Here's the drawing with two shaded views (mm, measured from the low corner). I have some questions. A direction names the side the tool comes from. Give positions to 0.01 mm unless a question says otherwise; leave off trailing zeros. Loops run counter-clockwise (first coordinate to the right, second up) from the corner with the lowest first, then second, coordinate; pieces in that order, holes last. Notation, with made-up numbers: (62.25, 29.5) -> (92.25, 29.5) arc R19 ccw to (92.25, 63.5) -> close; hole circle Ø1 at (1, 56). An arc over 180 degrees is marked (long way). Answer in a Markdown table with one row per item. Add a question column.
Item 1: If we section it at D-D (z = 1.25): Write out the boundary of the cut face in (x, y), then the cut area to 3 significant figures.
Item 2: If we section it at C-C (z = 9.25): Write out the boundary of the cut face in (x, y), then the cut area to 3 significant figures.
Item 3: If we section it at A-A (y = 5.5): Write out the boundary of the cut face in (x, z).
Item 4: If I drill on line 1 (Z direction, x = 9.5, y = 8.5); line 2 (Y direction, x = 9, z = 6); line 3 (X direction, y = 4, z = 2.5), over which ranges is the centre line in solid material (lowest first)?
Item 5: Which directions (+Z, -Z, +X, -X, +Y, -Y) give clear straight access to the entire face, cutting with the end or side of a thin tool? Please do the marked faces 1 and 2.
Item 6: For P1, Ø4, axis at x = 1.5, z = 10, coming from the -Y side; P2, Ø4, axis at y = 1.5, z = 6, coming from the +X side; P3, Ø4, axis at y = 8, z = 9.5, coming from the -X side, each with a flat end and sliding along its axis, tell me the tip position at first contact or that it passes through.
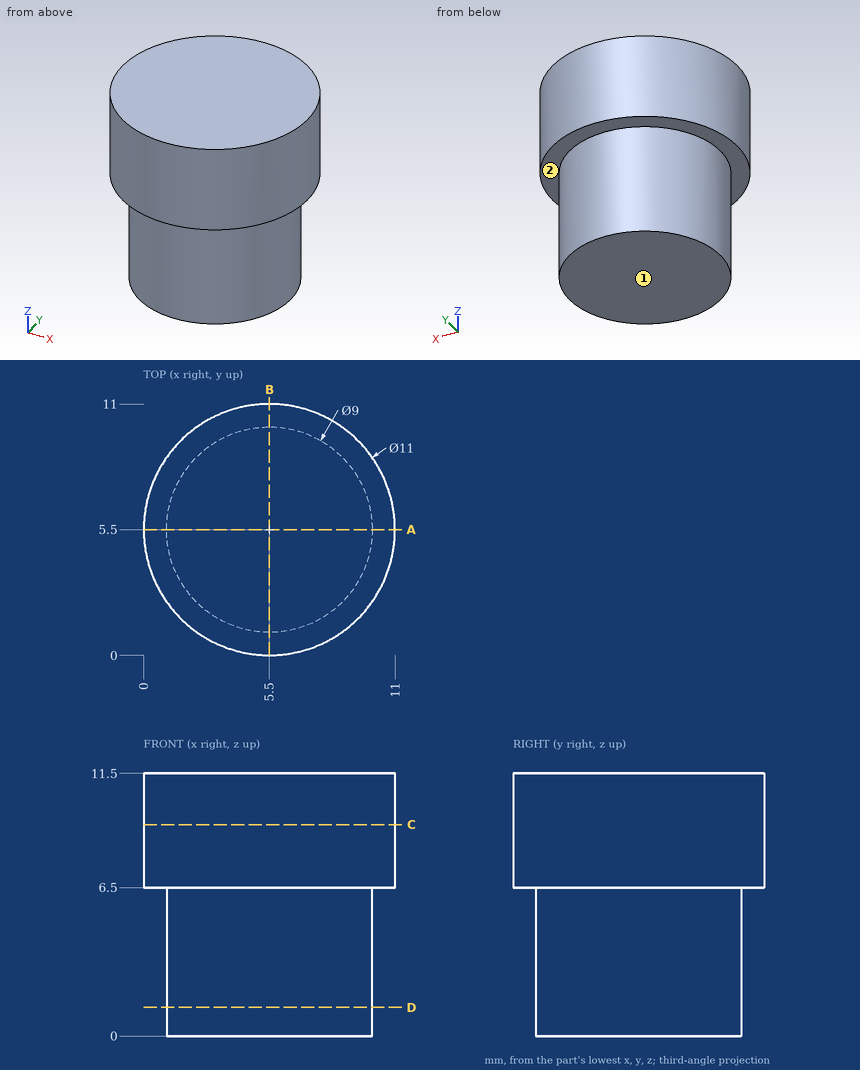
Recorded:
| question | item | result |
|---|---|---|
| 1 | outline | circle Ø9 at (5.5, 5.5) |
| 1 | area | 63.6 mm^2 |
| 2 | outline | circle Ø11 at (5.5, 5.5) |
| 2 | area | 95.0 mm^2 |
| 3 | outline | (0, 6.5) -> (1, 6.5) -> (1, 0) -> (10, 0) -> (10, 6.5) -> (11, 6.5) -> (11, 11.5) -> (0, 11.5) -> close |
| 4 | line 1 | z = 6.5 to 11.5 |
| 4 | line 2 | y = 2.67 to 8.33 |
| 4 | line 3 | x = 1.26 to 9.74 |
| 5 | face 1 | -Z, +X, -X, +Y, -Y |
| 5 | face 2 | -Z |
| 6 | P1 | stops at y = 0.38 |
| 6 | P2 | stops at x = 10.6 |
| 6 | P3 | stops at x = 0.02 |
